from build123d import *

# Parameters (mm, degrees)
BOSS_EXTRUDE1_DEPTH                = 6.35
F_10_32_TAPPED_HOLE1_AT_2_COUNT    = 2
F_10_32_TAPPED_HOLE1_AT_2_PITCH    = 19.05
F_5_16_0_3125_DIAMETER_HOLE1_D     = 7.9375
F_5_16_0_3125_DIAMETER_HOLE1_DEPTH = 10.668
F_5_16_0_3125_DIAMETER_HOLE1_TIP   = 2.38466558176563
CHAMFER1_SIZE                      = 1.5875
CUT_EXTRUDE1_DEPTH                 = 31.61859116615264
FILLET1_R                          = 6.35
CUT_EXTRUDE2_DEPTH                 = 31.61859116615264
FILLET2_R                          = 3.175
FILLET3_DEPTH                      = 6.35


with BuildPart() as part:
    # Sketch1 → Boss-Extrude1 (new body)
    with BuildSketch(Plane.XY):
        Polygon((-15.875000000000007, 25.400000000000006), (15.874999999999993, 25.400000000000006), (15.875, -25.39999999999999), (-15.875, -25.39999999999999), align=None)
    extrude(amount=BOSS_EXTRUDE1_DEPTH)

    # Sketch3 → #10-32 Tapped Hole1 (revolve, cut)
    with BuildSketch(Plane(origin=(-9.525000000000007, 25.400000000000006, 3.175000000000004), x_dir=(0, 0, 1), z_dir=(1, 0, 0))):
        Polygon((0, 0), (-2.66e-15, 10.865317848002352), (2.0192999999999977, 9.652), (2.0192999999999985, 4e-17), align=None)
    f_10_32_tapped_hole1 = revolve(axis=Axis((-9.525000000000007, 31.749999999999996, 3.175000000000004), (0, -1, 0)), mode=Mode.SUBTRACT)

    # #10-32 Tapped Hole1 at 2: #10-32 Tapped Hole1 ×2
    with Locations(*[(i * F_10_32_TAPPED_HOLE1_AT_2_PITCH, 0, 0) for i in range(1, F_10_32_TAPPED_HOLE1_AT_2_COUNT)]):
        add(f_10_32_tapped_hole1, mode=Mode.SUBTRACT)

    # 5/16 (0.3125) Diameter Hole1
    with Locations(Plane.XY.offset(6.35)):
        with Locations((0, 19.84375)):
            Hole(F_5_16_0_3125_DIAMETER_HOLE1_D / 2, depth=F_5_16_0_3125_DIAMETER_HOLE1_DEPTH)
            with Locations((0, 0, -(F_5_16_0_3125_DIAMETER_HOLE1_DEPTH + F_5_16_0_3125_DIAMETER_HOLE1_TIP / 2))):  # 118° drill point
                Cone(0, F_5_16_0_3125_DIAMETER_HOLE1_D / 2, F_5_16_0_3125_DIAMETER_HOLE1_TIP, mode=Mode.SUBTRACT)

    # Chamfer1
    chamfer1_edges = [part.edges().sort_by_distance(p)[0] for p in [
        (3.96875, 19.84375, 0),
        (3.96875, 19.84375, 6.35),
    ]]
    chamfer(chamfer1_edges, length=CHAMFER1_SIZE)

    # Sketch6 → Cut-Extrude1 (cut, through all)
    with BuildSketch(Plane.XY.offset(6.35)):
        with BuildLine():
            Line((-15.875000000000007, 17.462500000000006), (-15.875000000000007, 3.55e-15))
            Line((-15.875000000000007, 3.39e-15), (-8.92008318631283, 4.67e-15))
            ThreePointArc((-8.920083186312826, 3.5971e-13), (-10.722783415657506, 9.398268113531895), (-15.875000000000007, 17.462500000000006))
        make_face()
        with BuildLine():
            Line((-8.92008318631283, 4.67e-15), (-15.875000000000007, 3.39e-15))
            Line((-15.875000000000007, 3.55e-15), (-15.875000000000007, -17.462500000000006))
            ThreePointArc((-15.87500000000001, -17.46250000000001), (-10.722783415657375, -9.39826811353156), (-8.920083186312826, 3.5971e-13))
        make_face()
        with BuildLine():
            ThreePointArc((15.875000000000004, 17.462499999999984), (10.722783415657386, 9.39826811353155), (8.920083186312844, -3.4461e-13))
            Line((8.920083186312851, 7.94e-15), (15.875, 9.22e-15))
            Line((15.875000000000004, 1.066e-14), (15.875000000000004, 17.462499999999984))
        make_face()
        with BuildLine():
            Line((15.875, 9.22e-15), (8.920083186312851, 7.94e-15))
            ThreePointArc((8.920083186312844, -3.4461e-13), (10.722783415657513, -9.398268113531874), (15.875, -17.462499999999984))
            Line((15.875000000000004, -17.462499999999984), (15.875000000000004, 1.066e-14))
        make_face()
    extrude(amount=-CUT_EXTRUDE1_DEPTH, mode=Mode.SUBTRACT)

    # Fillet1
    fillet1_edges = [part.edges().sort_by_distance(p)[0] for p in [
        (15.875000000000002, -17.462499999999984, 3.175),
        (15.875000000000004, 17.462499999999984, 3.175),
        (-15.875000000000009, -17.46250000000001, 3.175),
        (-15.875000000000005, 17.462500000000006, 3.175),
    ]]
    fillet(fillet1_edges, radius=FILLET1_R)

    # Sketch7 → Cut-Extrude2 (cut, through all)
    with BuildSketch(Plane.XY.offset(6.35)):
        with BuildLine():
            Line((-8.92008318631281, -19.04999999999999), (8.920083186312835, -19.049999999999986))
            ThreePointArc((8.920083186312835, -19.049999999999986), (3.1152594113270133, -5.858453138165378), (3.7402393989355516, 8.540237346795667))
            ThreePointArc((3.7402393989355516, 8.540237346795667), (6.02e-15, 7.937499999999989), (-3.740239398935539, 8.540237346795662))
            ThreePointArc((-3.740239398935539, 8.540237346795662), (-3.1152594113270027, -5.858453138165384), (-8.92008318631281, -19.04999999999999))
        make_face()
    extrude(amount=-CUT_EXTRUDE2_DEPTH, mode=Mode.SUBTRACT)

    # Fillet2
    fillet2_edges = [part.edges().sort_by_distance(p)[0] for p in [
        (8.920083186312837, -19.049999999999986, 3.175),
        (-8.920083186312809, -19.04999999999999, 3.175),
    ]]
    fillet(fillet2_edges, radius=FILLET2_R)

    # Mirror1: #10-32 Tapped Hole1 across plane
    add(f_10_32_tapped_hole1.mirror(Plane.ZX), mode=Mode.SUBTRACT)

    # Mirror1 copy 1 sketch → Mirror1 copy 1 (revolve, cut)
    with BuildSketch(Plane(origin=(9.524999999999993, -25.400000000000006, 3.175000000000004), x_dir=(0, 0, 1), z_dir=(1, 0, 0))):
        Polygon((0, 0), (-2.66e-15, -10.865317848002352), (2.0192999999999977, -9.652), (2.0192999999999985, -4e-17), align=None)
    revolve(axis=Axis((9.524999999999993, -31.749999999999996, 3.175000000000004), (0, -1, 0)), mode=Mode.SUBTRACT)

    # Fillet3: read off the stored shape, not the designer's step
    # Fillet3 outline → Fillet3 (add)
    with BuildSketch(Plane.XY):
        with BuildLine():
            ThreePointArc((-3.740239399, 8.540237347), (-3.258151648, 6.574108997), (-2.902339746, 4.581254969))
            add(Edge.make_bspline(
                [(-2.902339746, 4.581254969), (-3.0109534907888404, 5.326116105248684), (-2.9047701826802874, 6.25797221448604), (-2.3933426209054938, 7.245588905615834), (-1.356695523735085, 7.937499999999987), (0, 7.9375)],
                knots=[0, 0, 0, 0, 0, 0, 0.5, 0.5, 0.5, 0.5, 0.5, 0.5], degree=5, weights=[1, 0.7711417009817829, 0.5994979767181202, 0.48506882720901173, 0.4278542524544575, 0.4278542524544575]))
            ThreePointArc((0, 7.9375), (-1.894246762, 8.089150123), (-3.740239399, 8.540237347))
        make_face()
        with BuildLine():
            ThreePointArc((3.740239399, 8.540237347), (1.894246748, 8.089150121), (-1.5e-08, 7.9375))
            add(Edge.make_bspline(
                [(-1.5e-08, 7.9375), (1.3566955237351, 7.937499999999984), (2.393342620905507, 7.245588905615829), (2.904770182680299, 6.257972214486036), (3.01095349078885, 5.326116105248681), (2.902339746, 4.581254969)],
                knots=[0.5, 0.5, 0.5, 0.5, 0.5, 0.5, 1, 1, 1, 1, 1, 1], degree=5, weights=[0.4278542524544575, 0.4278542524544575, 0.48506882720901173, 0.5994979767181202, 0.7711417009817829, 1]))
            ThreePointArc((2.902339746, 4.581254969), (3.258151648, 6.574108997), (3.740239399, 8.540237347))
        make_face()
    extrude(amount=FILLET3_DEPTH)


solid = part.part
Geometry check sheet. Reference: the model listing, model coordinates, mm. A direction names the side the tool comes from. Coordinates: 2 decimals unless noted, no trailing zeros. Write each loop counter-clockwise with the first axis right and the second up, starting at its lowest first coordinate (ties: lowest second). Pieces come first, ordered by that corner, then holes. Notation, with made-up numbers: (52.5, -37) -> (67.5, -37) arc R10 ccw to (67.5, -22) -> close; hole circle Ø9 at (-36.75, -17.75). An arc over 180 degrees is marked (long way). One line per question, with ' | ' between items.
1. Thickness scan on probe 1 along X at (y, z) = (17.5, 3.5); probe 2 along X at (y, z) = (0, 3); probe 3 along X at (y, z) = (-21, 4) (3 decimals). Record the ranges inside material, lowest first. Write a range as from..to.
Answers:
probe 1: x = -15.43..-11.52, -7.53..-3.2, 3.2..7.53, 11.52..15.43 | probe 2: x = -8.92..-2.57, 2.57..8.92 | probe 3: x = -15.875..-11.368, -7.682..7.682, 11.368..15.875
2. Cross-section at C-C on x = -2. State how many separate pieces and enclosed holes the cut face has, and give its area (3 significant figures).
Answers:
separate pieces: 3 | enclosed holes: 0 | area: 107 mm²
3. Draft check along X on faces 4 (the flat face through (-15.875, -23, 3)), 5 (the conical face through (-9.821, -14.745, 3.364)), 6 (the cylindrical face through (15.507, 17.701, 3.131)). Enter one of: +X half, -X half, draft (parallel to the pull), parting line (faces both ways), or undercut.
Answers:
face 4: -X half | face 5: undercut | face 6: +X half
4. Depth check by flat-ended pin: pin 1 Ø3.5 at (x, z) = (-9.525, 3.175) entering from +Y; pin 2 Ø5 at (x, y) = (11, 3.5) entering from +Z; pin 3 Ø10.5 at (x, y) = (0, 19.84) entering from +Z; pin 4 Ø2.5 at (x, z) = (-9.525, 3.175) entering from +Y. Enter the tip coordinate at first touch or a pass-through.
Answers:
pin 1: stops at y = 15.59 | pin 2: stops at z = 6.35 | pin 3: stops at z = 6.05 | pin 4: stops at y = 15.29
5. Cross-section at B-B on x = 14. Record the cut outline in (y, z), and give its area (3 significant figures).
Answers:
outline: (-25.4, 0) -> (-15.24, 0) -> (-15.24, 6.35) -> (-25.4, 6.35) -> close; (15.24, 0) -> (25.4, 0) -> (25.4, 6.35) -> (15.24, 6.35) -> close | area: 129 mm²
6. Set-up check for faces 1 (the cylindrical face through (3.016, -5.304, 3.219)), 2 (the cylindrical face through (11.316, -20.642, 4.107)), 3 (the cylindrical face through (15.527, -17.758, 3.131)): record each of +Z, -Z, +X, -X, +Y, -Y from which the full face is reachable in a straight line by a thin tool's end or side.
Answers:
face 1: +Z, -Z | face 2: -Y | face 3: +Z, -Z, +X
7. Cross-section at A-A on y = -2.5. Record the cut outline in (x, z), and give its area (3 significant figures).
Answers:
outline: (-9.04, 0) -> (-2.67, 0) -> (-2.67, 6.35) -> (-9.04, 6.35) -> close; (2.67, 0) -> (9.04, 0) -> (9.04, 6.35) -> (2.67, 6.35) -> close | area: 81.0 mm²
